Here's how the part is built. I have some questions about the finished solid (model axes, mm). A direction names the side the tool comes from. Give positions to 0.01 mm unless a question says otherwise; leave off trailing zeros. Order: outer loops, then holes, each group sorted by start corner. A loop starts at its lowest first (then second) coordinate and runs counter-clockwise, first axis right, second up. Notation, with made-up numbers: M 5.25,68.25 L 64.25,68.25 A14 ccw 64.25,86.25 Z; hole C -22,38 d1. An arc over 180 degrees is marked long. Use one line per item in the form item = value.
from build123d import *

# Parameters (mm, degrees)
SKETCH2_R           = 49.657
BOSS_EXTRUDE1_DEPTH = 6.35
SKETCH3_R           = 14.605
CUT_EXTRUDE1_DEPTH  = 6.35
SKETCH5_R           = 3.175
CUT_EXTRUDE2_DEPTH  = 6.35
CIRPATTERN1_COUNT   = 8


with BuildPart() as part:
    # Sketch2 → Boss-Extrude1 (new body)
    with BuildSketch(Plane(origin=(0, 0, 0), x_dir=(1, 0, 0), z_dir=(0, 1, 0))):
        with Locations(Location((0, 0, 0), (0, 0, 270))):
            Circle(SKETCH2_R)
    extrude(amount=BOSS_EXTRUDE1_DEPTH)

    # Sketch3 → Cut-Extrude1 (cut)
    with BuildSketch(Plane(origin=(0, 6.35, 0), x_dir=(1, 0, 0), z_dir=(0, 1, 0))):
        with Locations(Location((26.67, 0, 0), (0, 0, 270))):
            Circle(SKETCH3_R)
        with Locations(Location((-26.67, 0, 0), (0, 0, 270))):
            Circle(SKETCH3_R)
    extrude(amount=-CUT_EXTRUDE1_DEPTH, mode=Mode.SUBTRACT)

    # Sketch5 → Cut-Extrude2 (cut)
    with BuildSketch(Plane.XZ):
        with Locations(Location((0, 0, 0), (0, 0, 270))):
            Circle(SKETCH5_R)
    extrude(amount=-CUT_EXTRUDE2_DEPTH, mode=Mode.SUBTRACT)

    # Sketch8 → #6-32 Tapped Hole1 (revolve, cut)
    with BuildSketch(Plane(origin=(-19.002911201, 3.175, 45.877085946), x_dir=(0.9238795325112864, 0, 0.38268343236509056), z_dir=(0, 1, 0))):
        Polygon((0, 0), (0, 14.78269403), (1.35255, 13.97), (1.35255, 0), align=None)
    f_6_32_tapped_hole1 = revolve(axis=Axis((-21.432950996, 3.175, 51.743720977), (0.38268343236509056, 0, -0.9238795325112865)), mode=Mode.SUBTRACT)

    # CirPattern1: #6-32 Tapped Hole1 ×8 about axis
    cirpattern1_axis = Axis((0, -0.3175, 0), (0, 1, 0))
    for i in range(1, CIRPATTERN1_COUNT):
        add(f_6_32_tapped_hole1.rotate(cirpattern1_axis, i * 360 / CIRPATTERN1_COUNT), mode=Mode.SUBTRACT)


solid = part.part
Q1. I need wall thicknesses on L1, parallel to X at y = 2, z = 0 (3 decimals); L2, parallel to X at y = 4.5, z = 12; L3, parallel to X at y = 0.75, z = 1. Which ranges of each line are inside material? Lowest first, please.
Found:
L1 = -49.657 to -41.275, -12.065 to -3.175, 3.175 to 12.065, 41.275 to 49.657
L2 = -48.19 to -35, -18.34 to 18.34, 35 to 48.19
L3 = -49.65 to -41.24, -12.1 to -3.01, 3.01 to 12.1, 41.24 to 49.65
Q2. I want a section at A-A on z = 0. Write out the boundary of the cut face in (x, y) (3 decimals).
Found:
outline = M -49.657,0 L -41.275,0 L -41.275,6.35 L -49.657,6.35 Z; M -12.065,0 L -3.175,0 L -3.175,6.35 L -12.065,6.35 Z; M 3.175,0 L 12.065,0 L 12.065,6.35 L 3.175,6.35 Z; M 41.275,0 L 49.657,0 L 49.657,6.35 L 41.275,6.35 Z
Q3. On a 3-axis mill with a long thin cutter (end or side, diameter ignored), from which of +Z, -Z, +X, -X, +Y, -Y can I reach the whole of each face in a straight line? I mean faces 1 (the face through (12.412, 3.219, -3.166)), 2 (the face through (13.2, 3.26, -32.43)). Say none if no direction works.
Found:
face_1 = +Y, -Y
face_2 = none
Q4. I'm going to push flat-ended pins straight in: pin 1 Ø3 at (y, z) = (4.5, -21.5) entering from -X; pin 2 Ø2 at (x, y) = (19, 0.5) entering from -Z; pin 3 Ø3 at (y, z) = (5, -38.5) entering from -X; pin 4 Ø5 at (x, z) = (35.5, 12.5) entering from -Y. Where does each tip first touch, or does it pass through?
Found:
pin_1 = -45.45
pin_2 = -46.28
pin_3 = -33.12
pin_4 = 0
Q5. I want a section at D-D on x = 40. State how many separate pieces and enclosed holes the cut face has, then the cut area to 3 significant figures.
Found:
separate_pieces = 2
enclosed_holes = 2
area = 285 mm²
Q6. I want a section at B-B on x = 0. Write out the boundary of the cut face in (y, z) (3 decimals), then the cut area to 3 significant figures.
Found:
outline = M 0,-49.657 L 6.35,-49.657 L 6.35,-3.175 L 0,-3.175 Z; M 0,3.175 L 6.35,3.175 L 6.35,49.657 L 0,49.657 Z
area = 590 mm²
Q7. Thinking about a two-plate mould opening in Z: for faces 3 (the face through (-26.03, 3.22, -14.59)), 4 (the face through (33.56, 3.13, -36.6)), 5 (the face through (-10, 6.35, -1)), which applies, +Z half, -Z half, draft (parallel to the pull), parting line (faces both ways), or undercut?
Found:
face_3 = undercut
face_4 = parting line
face_5 = draft
Q8. I want a section at C-C on x = -26.67. Write out the boundary of the cut face in (y, z) (3 decimals), then the cut area to 3 significant figures.
Found:
outline = M 0,-41.887 L 6.35,-41.887 L 6.35,-14.605 L 0,-14.605 Z; M 0,14.605 L 6.35,14.605 L 6.35,41.887 L 0,41.887 Z
area = 346 mm²
